Design review of the part built by this model. Coordinates are the model's own, in mm. Coordinates: 2 decimals unless noted, no trailing zeros. Write each loop counter-clockwise with the first axis right and the second up, starting at its lowest first coordinate (ties: lowest second). Pieces come first, ordered by that corner, then holes.
Q1. Add section A-A, the plane x = -2.25. Give the boundary of the cut face in (y, z) (3 decimals), plus the area to 3 significant figures.
Q2. To check wall thickness, follow probe 1 along Y at (x, z) = (-1.25, -0.7) (3 decimals); probe 2 along Z at (x, y) = (-1.5, -0.75); probe 3 along Z at (x, y) = (-3.25, 1.6). State the ranges of each line that lie inside material, in increasing order.
Q3. The part is to be moulded in two halves that separate along Z. For faces 1 (the face through (-0.06, 0.06, 1.4)), 2 (the face through (0, 2.335, 0)), 3 (the face through (-3.91, -2.15, 1.25)), 4 (the face through (0.06, 1.15, -2.03)), say which applies: +Z half, -Z half, draft (parallel to the pull), parting line (faces both ways), or undercut.
from build123d import *

# Parameters (mm, degrees)
SKETCH1_R      = 1.4
EXTRUDE1_DEPTH = 4


# Read off the part's stored shape, not the designer's step: Cut-Extrude1
with BuildPart() as part:
    # Sketch1 → Extrude1 (new, symmetric)
    with BuildSketch(Plane(origin=(0, 0, 0), x_dir=(0, 0, -1), z_dir=(1, 0, 0))):
        Polygon((2.696225757, 0), (1.348112879, 2.335), (-1.348112879, 2.335), (-2.696225757, 0), (-1.348112879, -2.335), (1.348112879, -2.335), align=None)
        Circle(SKETCH1_R, mode=Mode.SUBTRACT)
    extrude(amount=EXTRUDE1_DEPTH, both=True)

    # Cut-Extrude1 outline → Cut-Extrude1 (revolve, cut)
    with BuildSketch(Plane.YX):
        Polygon((2.696225758, 4), (2.335, 4), (2.696225751, 3.791446215), align=None)
    cut_extrude1 = revolve(axis=Axis((0, 0, 0), (1, 0, 0)), mode=Mode.SUBTRACT)

    # Mirror1: Cut-Extrude1 across plane
    add(cut_extrude1.mirror(Plane(origin=(0, 0, 0), x_dir=(0, 0, 1), z_dir=(1, 0, 0))), mode=Mode.SUBTRACT)


solid = part.part
Here are the results:
1. outline: (-2.335, -1.348) - (0, -2.696) - (2.335, -1.348) - (2.335, 1.348) - (0, 2.696) - (-2.335, 1.348) - close; hole circle Ø2.8 at (0, 0)
1. area: 12.7 mm2
2. probe 1: y = -2.335 to -1.212, 1.212 to 2.335
2. probe 2: z = -2.26 to -1.18, 1.18 to 2.26
2. probe 3: z = -1.77 to 1.77
3. face 1: undercut
3. face 2: draft
3. face 3: +Z half
3. face 4: -Z half
